Check sheet for the modelled part. Datum: model origin and axes. Units: mm. A direction names the side the tool comes from. Round coordinates to 2 decimals unless told otherwise and drop trailing zeros. Write each loop counter-clockwise with the first axis right and the second up, starting at its lowest first coordinate (ties: lowest second). Pieces come first, ordered by that corner, then holes.
from build123d import *

# Parameters (mm, degrees)
SKETCH1_W           = 70
SKETCH1_H           = 120
BOSS_EXTRUDE1_DEPTH = 5
SKETCH2_W           = 20
SKETCH2_H           = 19
BOSS_EXTRUDE2_DEPTH = 18
SKETCH3_R           = 6
CUT_EXTRUDE1_DEPTH  = 109.415865998
CUT_EXTRUDE2_REACH  = 75.171
SKETCH4_R           = 1
SKETCH4_W           = 13
SKETCH4_H           = 23
SKETCH5_W           = 14
SKETCH5_H           = 5
BOSS_EXTRUDE3_DEPTH = 6
SKETCH6_R           = 1.55
CUT_EXTRUDE3_DEPTH  = 74.17103252


with BuildPart() as part:
    # Sketch1 → Boss-Extrude1 (new body)
    with BuildSketch(Plane.XY):
        Rectangle(SKETCH1_W, SKETCH1_H)
    extrude(amount=BOSS_EXTRUDE1_DEPTH)

    # Sketch2 → Boss-Extrude2 (add)
    with BuildSketch(Plane.XY.offset(5)):
        with Locations((-25, 30.5)):
            Rectangle(SKETCH2_W, SKETCH2_H)
        with Locations((25, 30.5)):
            Rectangle(SKETCH2_W, SKETCH2_H)
    extrude(amount=BOSS_EXTRUDE2_DEPTH)

    # Sketch3 → Cut-Extrude1 (cut, through all)
    with BuildSketch(Plane(origin=(0, 40, 0), x_dir=(1, 0, 0), z_dir=(0, 1, 0))):
        with Locations(Location((-25, -14, 0), (0, 0, 180))):
            Circle(SKETCH3_R)
        with Locations(Location((25, -14, 0), (0, 0, 180))):
            Circle(SKETCH3_R)
    extrude(amount=-CUT_EXTRUDE1_DEPTH, mode=Mode.SUBTRACT)

    # Sketch4 → Cut-Extrude2 (cut, up to next)
    with BuildSketch(Plane(origin=(0, 0, 0), x_dir=(-1, 0, 0), z_dir=(0, 0, -1)), mode=Mode.PRIVATE) as cut_extrude2_sk1:
        with Locations((0, -11.2)):
            Circle(SKETCH4_R)
    cut_extrude2_tool1 = extrude(cut_extrude2_sk1.sketch, amount=-CUT_EXTRUDE2_REACH, mode=Mode.PRIVATE) & part.part
    # Sketch4 → Cut-Extrude2 (cut, up to next)
    with BuildSketch(Plane(origin=(0, 0, 0), x_dir=(-1, 0, 0), z_dir=(0, 0, -1)), mode=Mode.PRIVATE) as cut_extrude2_sk2:
        with Locations((0, -38.8)):
            Circle(SKETCH4_R)
    cut_extrude2_tool2 = extrude(cut_extrude2_sk2.sketch, amount=-CUT_EXTRUDE2_REACH, mode=Mode.PRIVATE) & part.part
    # Sketch4 → Cut-Extrude2 (cut, up to next)
    with BuildSketch(Plane(origin=(0, 0, 0), x_dir=(-1, 0, 0), z_dir=(0, 0, -1)), mode=Mode.PRIVATE) as cut_extrude2_sk3:
        with Locations((0, -25)):
            Rectangle(SKETCH4_W, SKETCH4_H)
    cut_extrude2_tool3 = extrude(cut_extrude2_sk3.sketch, amount=-CUT_EXTRUDE2_REACH, mode=Mode.PRIVATE) & part.part
    add(cut_extrude2_tool1.solids().sort_by_distance((0, -11.2, 0))[0], mode=Mode.SUBTRACT)
    add(cut_extrude2_tool2.solids().sort_by_distance((0, -38.8, 0))[0], mode=Mode.SUBTRACT)
    add(cut_extrude2_tool3.solids().sort_by_distance((0, -25, 0))[0], mode=Mode.SUBTRACT)

    # Sketch5 → Boss-Extrude3 (add)
    with BuildSketch(Plane.XY.offset(5)):
        with Locations((-7, 45.5)):
            Rectangle(SKETCH5_W, SKETCH5_H)
    extrude(amount=BOSS_EXTRUDE3_DEPTH)

    # Sketch6 → Cut-Extrude3 (cut, through all)
    with BuildSketch(Plane(origin=(0, 0, 0), x_dir=(-1, 0, 0), z_dir=(0, 0, -1))):
        with Locations((-11, -7)):
            Circle(SKETCH6_R)
        with Locations((-11, -43)):
            Circle(SKETCH6_R)
    extrude(amount=-CUT_EXTRUDE3_DEPTH, mode=Mode.SUBTRACT)


solid = part.part
1. Sectioned sample at D-D, the plane y = 25. Enter the section's corners in (x, z), plus the area to 3 significant figures.
2. Release check for a two-part mould opening along X. For faces 6 (the flat face through (0, 45, 8)), 7 (the flat face through (-7, 43, 8)), 8 (the cylindrical face through (11.336, -44.513, 2.465)) record: released by +X, released by -X, zero draft, split by the parting line, or undercut.
3. Sectioned sample at B-B, the plane z = 21.5. Enter the section's corners in (x, y), plus the area to 3 significant figures.
4. Scan lines: line 1 along Y through (x, z) = (0, 3.6); line 2 along Z through (x, y) = (-25, 33); line 3 along Y through (x, z) = (11, 2.85). Record each from-to range of solid material in increasing order.
5. Sectioned sample at A-A, the plane y = -7. Enter the section's corners in (x, z), plus the area to 4 significant figures.
6. Sectioned sample at C-C, the plane x = 11. Enter the section's corners in (y, z).
7. Go/stop test with flat-tipped pins: pin 1 (9 mm diameter, centred on x = 22, z = 14, fed in from -Y); pin 2 (7 mm diameter, centred on x = -25, z = 14, fed in from -Y); pin 3 (8 mm diameter, centred on x = -6, z = 14.5, fed in from -Y); pin 4 (2.5 mm diameter, centred on x = 0, y = -38.8, fed in from +Z). Record where each tip stops, or that it passes through.
8. Set-up check for faces 1 (the flat face through (35, 12, 4)), 2 (the flat face through (-30, 21, 10)), 3 (the flat face through (-15, 30, 14)), 4 (the flat face through (0, -36.5, 2)), 5 (the flat face through (20, 40, 10)): record each of +Z, -Z, +X, -X, +Y, -Y from which the full face is reachable in a straight line by a thin tool's end or side.
Computed values:
1. outline: (-35, 0) - (35, 0) - (35, 23) - (15, 23) - (15, 5) - (-15, 5) - (-15, 23) - (-35, 23) - close; hole circle Ø12 at (-25, 14); hole circle Ø12 at (25, 14)
1. area: 844 mm2
2. face 6: released by +X
2. face 7: zero draft
2. face 8: undercut
3. outline: (-35, 21) - (-15, 21) - (-15, 40) - (-35, 40) - close; (15, 21) - (35, 21) - (35, 40) - (15, 40) - close
3. area: 760 mm2
4. line 1: y = -60 to -39.8, -37.8 to -36.5, -13.5 to -12.2, -10.2 to 60
4. line 2: z = 0 to 8, 20 to 23
4. line 3: y = -60 to -44.55, -41.45 to -8.55, -5.45 to 60
5. outline: (-35, 0) - (9.45, 0) - (9.45, 5) - (-35, 5) - close; (12.55, 0) - (35, 0) - (35, 5) - (12.55, 5) - close
5. area: 334.5 mm2
6. outline: (-60, 0) - (-44.55, 0) - (-44.55, 5) - (-60, 5) - close; (-41.45, 0) - (-8.55, 0) - (-8.55, 5) - (-41.45, 5) - close; (-5.45, 0) - (60, 0) - (60, 5) - (-5.45, 5) - close
7. pin 1: stops at y = 21
7. pin 2: passes through
7. pin 3: stops at y = 43
7. pin 4: stops at z = 5
8. face 1: +Z, -Z, +X, +Y, -Y
8. face 2: +Z, +X, -X, -Y
8. face 3: +Z, +Y, -Y
8. face 4: +Z, -Z
8. face 5: +Z, +X, -X, +Y
